Drawing for the job (mm, zero at the part's lowest x, y, z). A direction names the side the tool comes from. Round coordinates to 2 decimals unless told otherwise and drop trailing zeros. Order: outer loops, then holes, each group sorted by start corner. A loop starts at its lowest first (then second) coordinate and runs counter-clockwise, first axis right, second up. Notation, with made-up numbers: M -36.75,6.25 L -13.75,6.25 A21 ccw -13.75,36.25 Z; hole C 79,-10 d4. An arc over 180 degrees is marked long. One line per item, written item: value. Start each with the question number.
Item 1: Band-saw the part on B-B, the plane z = 1.5. Write the cut outline in (x, y) (3 decimals), then the cut area to 3 significant figures.
Item 2: Probe L1, parallel to X at y = 8.6, z = 1.5 (3 decimals); L2, parallel to Y at x = 13.25, z = 2.55; L3, parallel to X at y = 10, z = 2.4. List the from-to ranges inside material, lowest first.
Item 3: Two-plate mould, pull along X, no slides. Class the marked faces 4, 5 and 6: +X half, -X half, draft (parallel to the pull), parting line (faces both ways), or undercut.
Item 4: Tool access for the marked faces 1, 2 and 3: list every direction of +Z, -Z, +X, -X, +Y, -Y with a clear straight run to the whole face (end or side of a thin tool).
Item 5: Band-saw the part on C-C, the plane x = 6.75. Write the cut outline in (y, z), then the cut area to 4 significant figures.
Item 6: Band-saw the part on A-A, the plane y = 9. Write the cut outline in (x, z) (3 decimals), then the cut area to 3 significant figures.
Item 7: Pin check, flat tip, straight feed: pin 1 (1.5 mm diameter, centred on x = 13.5, z = 1.5, fed in from +Y). Stop position of the tip, or through.
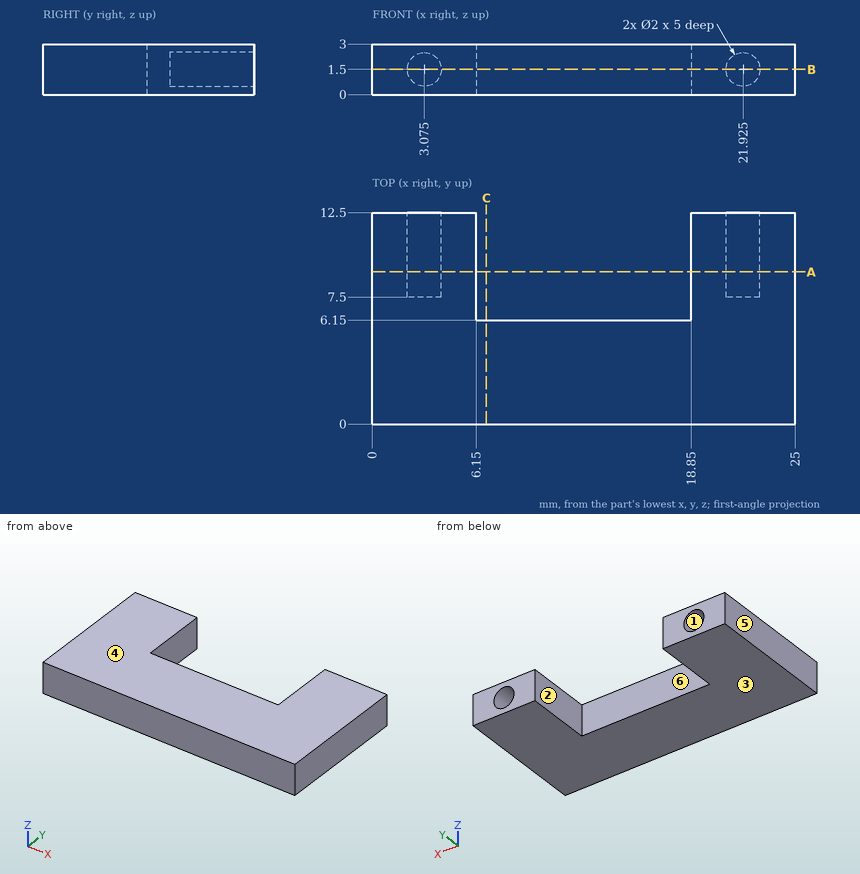
Output:
1. outline: M 0,0 L 25,0 L 25,12.5 L 22.925,12.5 L 22.925,7.5 L 20.925,7.5 L 20.925,12.5 L 18.85,12.5 L 18.85,6.15 L 6.15,6.15 L 6.15,12.5 L 4.075,12.5 L 4.075,7.5 L 2.075,7.5 L 2.075,12.5 L 0,12.5 Z
1. area: 212 mm²
2. L1: x = 0 to 2.075, 4.075 to 6.15, 18.85 to 20.925, 22.925 to 25
2. L2: y = 0 to 6.15
2. L3: x = 0 to 2.64, 3.51 to 6.15, 18.85 to 21.49, 22.36 to 25
3. face 4: draft
3. face 5: -X half
3. face 6: undercut
4. face 1: +Y
4. face 2: +Z, -Z, +Y
4. face 3: -Z, +X, -X, +Y, -Y
5. outline: M 0,0 L 6.15,0 L 6.15,3 L 0,3 Z
5. area: 18.45 mm²
6. outline: M 0,0 L 6.15,0 L 6.15,3 L 0,3 Z; M 18.85,0 L 25,0 L 25,3 L 18.85,3 Z; hole C 3.075,1.5 d2; hole C 21.925,1.5 d2
6. area: 30.6 mm²
7. pin 1: stops at y = 6.15
